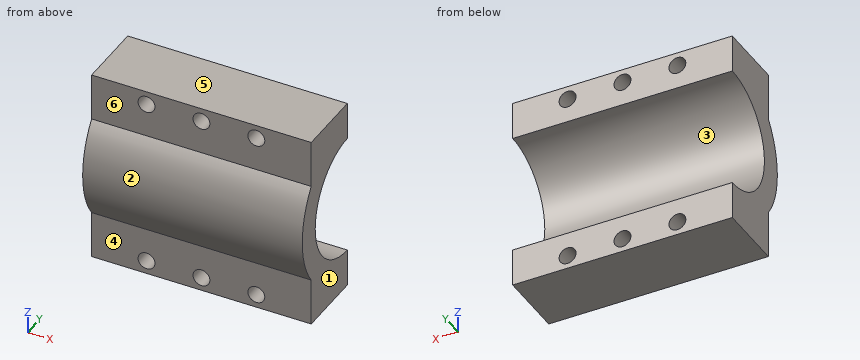
```python
from build123d import *

# Parameters (mm, degrees)
SKETCH1_W           = 65
SKETCH1_H           = 58
SKETCH1_R           = 2.5
BOSS_EXTRUDE1_DEPTH = 25
SKETCH2_R           = 17.825
CUT_EXTRUDE1_DEPTH  = 76.43871685


with BuildPart() as part:
    # Sketch1 → Boss-Extrude1 (new body)
    with BuildSketch(Plane(origin=(0, 0, 0), x_dir=(1, 0, 0), z_dir=(0, 1, 0))):
        Rectangle(SKETCH1_W, SKETCH1_H)
        with Locations(Location((-16.25, 25, 0), (0, 0, 270))):
            Circle(SKETCH1_R, mode=Mode.SUBTRACT)
        with Locations(Location((16.25, 25, 0), (0, 0, 270))):
            Circle(SKETCH1_R, mode=Mode.SUBTRACT)
        with Locations(Location((16.25, -25, 0), (0, 0, 90))):
            Circle(SKETCH1_R, mode=Mode.SUBTRACT)
        with Locations(Location((-16.25, -25, 0), (0, 0, 90))):
            Circle(SKETCH1_R, mode=Mode.SUBTRACT)
        with Locations(Location((0, 25, 0), (0, 0, 270))):
            Circle(SKETCH1_R, mode=Mode.SUBTRACT)
        with Locations(Location((0, -25, 0), (0, 0, 270))):
            Circle(SKETCH1_R, mode=Mode.SUBTRACT)
    extrude(amount=BOSS_EXTRUDE1_DEPTH)

    # Sketch2 → Cut-Extrude1 (cut, through all)
    with BuildSketch(Plane(origin=(32.5, 0, 0), x_dir=(0, 0, -1), z_dir=(1, 0, 0))):
        with Locations((0, 25)):
            Circle(SKETCH2_R)
        with BuildLine():
            Line((-14.963830053, 4.972923575), (-29, 4.972923575))
            Line((-29, 4.972923575), (-29, -6.793967085))
            Line((-29, -6.793967085), (29, -6.793967085))
            Line((29, -6.793967085), (29, 4.972923575))
            Line((29, 4.972923575), (14.963830053, 4.972923575))
            ThreePointArc((14.963830053, 4.972923575), (0, 0), (-14.963830053, 4.972923575))
        make_face()
    extrude(amount=-CUT_EXTRUDE1_DEPTH, mode=Mode.SUBTRACT)


solid = part.part
```
Verification items for the finished model (mm, model axes). Face numbers are marked on the shaded views. A direction names the side the tool comes from. Coordinates: 2 decimals unless noted, no trailing zeros. Loops run counter-clockwise (first coordinate to the right, second up) from the corner with the lowest first, then second, coordinate; pieces in that order, holes last. Notation, with made-up numbers: (25.5, 27.25) -> (38.5, 27.25) arc R23 cw to (38.5, 57.25) -> close; hole circle Ø10 at (54, 79.5). An arc over 180 degrees is marked (long way). Answer in a Markdown table with one row per item. Add a question column.
1. Section check B-B, the plane y = 22.75. Enter the section's corners in (x, z).
2. Section check C-C, the plane z = -25. Enter the section's corners in (x, y).
3. Section check D-D, the plane y = 13. Enter the section's corners in (x, z), then the cut area to 3 significant figures.
4. Section check A-A, the plane x = -16.25. Enter the section's corners in (y, z) (3 decimals), then the cut area to 3 significant figures.
5. Access from +Z, -Z, +X, -X, +Y, -Y to the whole of each face (thin tool, end or side, straight path). Record for the marked faces 4, 5 and 6.
6. Material ranges on probe 1 along X at (y, z) = (11.5, 25); probe 2 along Z at (x, y) = (-16, 15.75); probe 3 along Z at (x, y) = (-16.25, 9.75), recorded low to high. Write a range as [from, to].
7. Draft check along Z on the marked faces 1, 2 and 3. Enter one of: +Z half, -Z half, draft (parallel to the pull), parting line (faces both ways), or undercut.
8. Depth check by flat-ended pin: P1, Ø6.5, axis at x = -16.25, z = -25, coming from the -Y side; P2, Ø3, axis at x = -25.5, z = 15.5, coming from the -Y side; P3, Ø1, axis at x = 13, z = 8, coming from the +Y side. Enter the tip coordinate at first touch or a pass-through.
Derived:
| question | item | result |
|---|---|---|
| 1 | outline | (-32.5, -29) -> (32.5, -29) -> (32.5, -17.68) -> (-32.5, -17.68) -> close; (-32.5, 17.68) -> (32.5, 17.68) -> (32.5, 29) -> (-32.5, 29) -> close; hole circle Ø5 at (-16.25, -25); hole circle Ø5 at (-16.25, 25); hole circle Ø5 at (0, -25); hole circle Ø5 at (0, 25); hole circle Ø5 at (16.25, -25); hole circle Ø5 at (16.25, 25) |
| 2 | outline | (-32.5, 4.97) -> (-18.75, 4.97) -> (-18.75, 25) -> (-32.5, 25) -> close; (-13.75, 4.97) -> (-2.5, 4.97) -> (-2.5, 25) -> (-13.75, 25) -> close; (2.5, 4.97) -> (13.75, 4.97) -> (13.75, 25) -> (2.5, 25) -> close; (18.75, 4.97) -> (32.5, 4.97) -> (32.5, 25) -> (18.75, 25) -> close |
| 3 | outline | (-32.5, -29) -> (32.5, -29) -> (32.5, -13.18) -> (-32.5, -13.18) -> close; (-32.5, 13.18) -> (32.5, 13.18) -> (32.5, 29) -> (-32.5, 29) -> close; hole circle Ø5 at (-16.25, -25); hole circle Ø5 at (-16.25, 25); hole circle Ø5 at (0, -25); hole circle Ø5 at (0, 25); hole circle Ø5 at (16.25, -25); hole circle Ø5 at (16.25, 25) |
| 3 | area | 1,940 mm² |
| 4 | outline | (4.973, -29) -> (25, -29) -> (25, -27.5) -> (4.973, -27.5) -> close; (4.973, -22.5) -> (25, -22.5) -> (25, -17.825) arc R17.825 cw to (25, 17.825) -> (25, 22.5) -> (4.973, 22.5) -> (4.973, 14.964) arc R25 ccw to (4.973, -14.964) -> close; (4.973, 27.5) -> (25, 27.5) -> (25, 29) -> (4.973, 29) -> close |
| 4 | area | 564 mm² |
| 5 | face 4 | -Z, +X, -X, -Y |
| 5 | face 5 | +Z, +X, -X, +Y, -Y |
| 5 | face 6 | +Z, +X, -X, -Y |
| 6 | probe 1 | x = [-32.5, -18.75], [-13.75, -2.5], [2.5, 13.75], [18.75, 32.5] |
| 6 | probe 2 | z = [-29, -27.49], [-22.51, -15.24], [15.24, 22.51], [27.49, 29] |
| 6 | probe 3 | z = [-29, -27.5], [-22.5, -9.23], [9.23, 22.5], [27.5, 29] |
| 7 | face 1 | draft |
| 7 | face 2 | parting line |
| 7 | face 3 | undercut |
| 8 | P1 | stops at y = 4.97 |
| 8 | P2 | stops at y = 4.29 |
| 8 | P3 | stops at y = 9.33 |
